from build123d import *

# Parameters (mm, degrees)
SKETCH_1_W          = 100
SKETCH_1_H          = 50
EXTRUDE_1_DEPTH     = 12
SKETCH_2_R          = 4
CUT_EXTRUDE_1_DEPTH = 58.175169436
SKETCH_3_R          = 15
EXTRUDE_2_DEPTH     = 33
SKETCH_4_R          = 7.5
CUT_EXTRUDE_2_DEPTH = 72.763500472
SKETCH_5_W          = 8
SKETCH_5_H          = 30
CUT_EXTRUDE_3_DEPTH = 5
FILLET_2_R          = 10
FILLET_3_R          = 10
RIB_30_REACH        = 73.764
SKETCH_11_WALL_W    = 185.838289686
SKETCH_11_WALL_H    = 8
RIB_31_REACH        = 73.764
SKETCH_15_WALL_W    = 185.838289686
SKETCH_15_WALL_H    = 8
SKETCH_16_R         = 4
CUT_EXTRUDE_4_DEPTH = 79.262379212


with BuildPart() as part:
    # Sketch 1 → Extrude 1 (new body)
    with BuildSketch(Plane(origin=(0, 0, 0), x_dir=(1, 0, 0), z_dir=(0, 1, 0))):
        Rectangle(SKETCH_1_W, SKETCH_1_H)
    extrude(amount=EXTRUDE_1_DEPTH)

    # Sketch 2 → Cut-Extrude 1 (cut, through all)
    with BuildSketch(Plane(origin=(0, 12, 0), x_dir=(1, 0, 0), z_dir=(0, 1, 0))):
        with Locations(Location((-40, -20, 0), (0, 0, 270))):
            Circle(SKETCH_2_R)
        with Locations(Location((-40, 20, 0), (0, 0, 90))):
            Circle(SKETCH_2_R)
        with Locations(Location((40, -20, 0), (0, 0, 90))):
            Circle(SKETCH_2_R)
        with Locations(Location((40, 20, 0), (0, 0, 270))):
            Circle(SKETCH_2_R)
    extrude(amount=-CUT_EXTRUDE_1_DEPTH, mode=Mode.SUBTRACT)

    # Sketch 3 → Extrude 2 (add)
    with BuildSketch(Plane(origin=(0, 12, 0), x_dir=(1, 0, 0), z_dir=(0, 1, 0))):
        with Locations(Location((0, 0, 0), (0, 0, 270))):
            Circle(SKETCH_3_R)
    extrude(amount=EXTRUDE_2_DEPTH)

    # Sketch 4 → Cut-Extrude 2 (cut, through all)
    with BuildSketch(Plane(origin=(0, 45, 0), x_dir=(1, 0, 0), z_dir=(0, 1, 0))):
        with Locations(Location((0, 0, 0), (0, 0, 270))):
            Circle(SKETCH_4_R)
    extrude(amount=-CUT_EXTRUDE_2_DEPTH, mode=Mode.SUBTRACT)

    # Sketch 5 → Cut-Extrude 3 (cut)
    with BuildSketch(Plane(origin=(0, 45, 0), x_dir=(1, 0, 0), z_dir=(0, 1, 0))):
        Rectangle(SKETCH_5_W, SKETCH_5_H)
    extrude(amount=-CUT_EXTRUDE_3_DEPTH, mode=Mode.SUBTRACT)

    # Fillet 2
    fillet_2_edges = [part.edges().sort_by_distance(p)[0] for p in [
        (-50, 6, 25),
        (-50, 6, -25),
    ]]
    fillet(fillet_2_edges, radius=FILLET_2_R)

    # Fillet 3
    fillet_3_edges = [part.edges().sort_by_distance(p)[0] for p in [
        (50, 6, -25),
        (50, 6, 25),
    ]]
    fillet(fillet_3_edges, radius=FILLET_3_R)

    # Sketch 11 wall → Rib 30 (add, up to next)
    with BuildSketch(Plane(origin=(-32.5, 22, 0), x_dir=(0.868243142124, 0.496138938357, 0), z_dir=(-0.496138938357, 0.868243142124, 0)), mode=Mode.PRIVATE) as rib_30_sk1:
        Rectangle(SKETCH_11_WALL_W, SKETCH_11_WALL_H)
    rib_30_tool1 = extrude(rib_30_sk1.sketch, amount=-RIB_30_REACH, mode=Mode.PRIVATE) - part.part
    add(rib_30_tool1.solids().sort_by_distance((-32.5, 22, 0))[0])

    # Sketch 15 wall → Rib 31 (add, up to next)
    with BuildSketch(Plane(origin=(32.5, 22, 0), x_dir=(-0.868243142124, 0.496138938357, 0), z_dir=(-0.496138938357, -0.868243142124, 0)), mode=Mode.PRIVATE) as rib_31_sk1:
        Rectangle(SKETCH_15_WALL_W, SKETCH_15_WALL_H)
    rib_31_tool1 = extrude(rib_31_sk1.sketch, amount=RIB_31_REACH, mode=Mode.PRIVATE) - part.part
    add(rib_31_tool1.solids().sort_by_distance((32.5, 22, 0))[0])

    # Sketch 16 → Cut-Extrude 4 (cut, through all)
    with BuildSketch(Plane.XY.offset(15)):
        with Locations((0, 22)):
            Circle(SKETCH_16_R)
    extrude(amount=-CUT_EXTRUDE_4_DEPTH, mode=Mode.SUBTRACT)


solid = part.part
Geometry check sheet. Reference: the model listing, model coordinates, mm. A direction names the side the tool comes from. Round coordinates to 2 decimals unless told otherwise and drop trailing zeros. Write each loop counter-clockwise with the first axis right and the second up, starting at its lowest first coordinate (ties: lowest second). Pieces come first, ordered by that corner, then holes. Notation, with made-up numbers: (35, -40) - (75, -40) arc R11 ccw to (75, -27) - close; hole circle Ø2 at (62, 32). An arc over 180 degrees is marked (long way). One line per item, written item: value.
1. Scan lines: L1, parallel to X at y = 3.5, z = -20; L2, parallel to Z at x = 0, y = 10; L3, parallel to Y at x = 0, z = -12. Record each from-to range of solid material in increasing order.
The answers:
L1: x = -48.66 to -44, -36 to 36, 44 to 48.66
L2: z = -25 to -7.5, 7.5 to 25
L3: y = 0 to 18, 26 to 40
2. Depth check by flat-ended pin: pin 1 Ø6 at (y, z) = (19.5, -11.5) entering from -X; pin 2 Ø2.5 at (y, z) = (42, 12.5) entering from +X; pin 3 Ø1 at (x, y) = (-6, 35.5) entering from +Z; pin 4 Ø7 at (x, z) = (-40, 20) entering from +Y. Enter the tip coordinate at first touch or a pass-through.
The answers:
pin 1: stops at x = -12.36
pin 2: stops at x = 9.92
pin 3: stops at z = 13.96
pin 4: passes through
3. Mould release check, pull along X, two halves, no side actions. Record for faces 4 (the face through (-1, 12, -17)), 5 (the face through (4, 43, 10)), 6 (the face through (46.99, 6.08, -22.15)): released by +X, released by -X, zero draft, split by the parting line, or undercut.
The answers:
face 4: zero draft
face 5: undercut
face 6: released by +X
4. Cross-section at C-C on y = 30. Record the boundary of the cut face in (x, z).
The answers:
outline: (-18.5, -4) - (-14.46, -4) arc R15 ccw to (14.46, -4) - (18.5, -4) - (18.5, 4) - (14.46, 4) arc R15 ccw to (-14.46, 4) - (-18.5, 4) - close; hole circle Ø15 at (0, 0)
5. Cross-section at B-B on z = 0. Record the boundary of the cut face in (x, y).
The answers:
outline: (-50, 0) - (-7.5, 0) - (-7.5, 45) - (-15, 45) - (-15, 32) - (-50, 12) - close; (7.5, 0) - (50, 0) - (50, 12) - (15, 32) - (15, 45) - (7.5, 45) - close
6. Set-up check for faces 1 (the face through (-4, 43, -10)), 2 (the face through (26, 20, -4)), 3 (the face through (-26, 20, -4)): record each of +Z, -Z, +X, -X, +Y, -Y from which the full face is reachable in a straight line by a thin tool's end or side.
The answers:
face 1: +Z, -Z, +Y
face 2: -Z, +X, +Y
face 3: -Z, -X, +Y
7. Cross-section at D-D on z = -9. Record the boundary of the cut face in (x, y), and give its area (3 significant figures).
The answers:
outline: (-50, 0) - (50, 0) - (50, 12) - (12, 12) - (12, 45) - (4, 45) - (4, 40) - (-4, 40) - (-4, 45) - (-12, 45) - (-12, 12) - (-50, 12) - close; hole circle Ø8 at (0, 22)
area: 1,900 mm^2
8. Cross-section at A-A on y = 22. Record the boundary of the cut face in (x, z).
The answers:
outline: (-32.5, -4) - (-14.46, -4) arc R15 ccw to (-4, -14.46) - (-4, -6.34) arc R7.5 cw to (-4, 6.34) - (-4, 14.46) arc R15 ccw to (-14.46, 4) - (-32.5, 4) - close; (4, -14.46) arc R15 ccw to (14.46, -4) - (32.5, -4) - (32.5, 4) - (14.46, 4) arc R15 ccw to (4, 14.46) - (4, 6.34) arc R7.5 cw to (4, -6.34) - close
